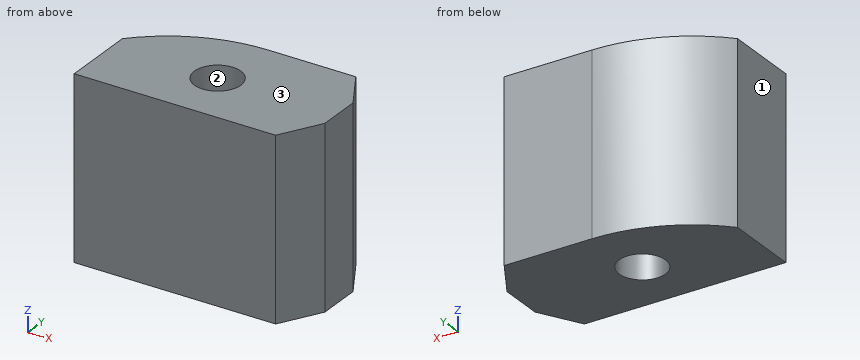
```python
from build123d import *

# Parameters (mm, degrees)
SKETCH1_R           = 7.5
BOSS_EXTRUDE2_DEPTH = 58


with BuildPart() as part:
    # Sketch1 → Boss-Extrude2 (new body)
    with BuildSketch(Plane.XY):
        with BuildLine():
            Line((-34, 5), (-34, -19))
            Line((-34, -19), (31, -19))
            Line((31, -19), (38.5, -6.009618943))
            Line((38.5, -6.009618943), (38.5, 8.009618943))
            Line((38.5, 8.009618943), (31, 21))
            Line((31, 21), (2.66060556, 21))
            ThreePointArc((2.66060556, 21), (-17.33939444, 16.82575695), (-34, 5))
        make_face()
        with Locations(Location((0, 0, 0), (0, 0, 180))):
            Circle(SKETCH1_R, mode=Mode.SUBTRACT)
    extrude(amount=BOSS_EXTRUDE2_DEPTH)


solid = part.part
```
Part model, mm, in its own coordinate system. Face numbers are marked on the shaded views. Round coordinates to 2 decimals unless told otherwise and drop trailing zeros. Loops run counter-clockwise (first coordinate to the right, second up) from the corner with the lowest first, then second, coordinate; pieces in that order, holes last. Notation, with made-up numbers: (-16, 61) -> (17, 61) arc R23 cw to (17, 76) -> close; hole circle Ø8 at (44, 42). An arc over 180 degrees is marked (long way). Use CSV: the item, a comma, the result in double quotes. Start each with the question number.
1) Cut at C-C, the plane x = -5. Write the cut outline in (y, z).
2) Cut at A-A, the plane y = 0. Write the cut outline in (x, z).
3) Drop flat-ended pins along their axis: P1, Ø13.5, axis at x = 0, y = 0, coming from the -Z side (1 decimal); P2, Ø5, axis at y = 11.5, z = 9, coming from the +X side. Give the stop position or say it passes through.
4) Cut at D-D, the plane y = -13. Write the cut outline in (x, z), plus the area to 3 significant figures.
5) Pull direction X, two halves, no side cores. Call the marked faces 1, 2 and 3: +X half, -X half, draft (parallel to the pull), parting line (faces both ways), or undercut.
6) Cut at B-B, the plane z = 9.5. Write the cut outline in (x, y), plus the area to 3 significant figures.
7) Wall check: L1, parallel to Y at x = 0, z = 12.5; L2, parallel to X at y = 5, z = 12.5; L3, parallel to X at y = 3.5, z = 26. Give the ranges that are in metal, low to high. Write a range as [from, to].
Determined:
1,outline,"(-19, 0) -> (-5.59, 0) -> (-5.59, 58) -> (-19, 58) -> close; (5.59, 0) -> (20.41, 0) -> (20.41, 58) -> (5.59, 58) -> close"
2,outline,"(-34, 0) -> (-7.5, 0) -> (-7.5, 58) -> (-34, 58) -> close; (7.5, 0) -> (38.5, 0) -> (38.5, 58) -> (7.5, 58) -> close"
3,P1,"passes through"
3,P2,"stops at x = 37.93"
4,outline,"(-34, 0) -> (34.46, 0) -> (34.46, 58) -> (-34, 58) -> close"
4,area,"3,970 mm2"
5,face 1,"-X half"
5,face 2,"undercut"
5,face 3,"draft"
6,outline,"(-34, -19) -> (31, -19) -> (38.5, -6.01) -> (38.5, 8.01) -> (31, 21) -> (2.66, 21) arc R50 ccw to (-34, 5) -> close; hole circle Ø15 at (0, 0)"
6,area,"2,440 mm2"
7,L1,"y = [-19, -7.5], [7.5, 20.93]"
7,L2,"x = [-34, -5.59], [5.59, 38.5]"
7,L3,"x = [-34, -6.63], [6.63, 38.5]"
